Geometry: final body of the model. Coordinates: model frame, mm. A direction names the side the tool comes from. Round coordinates to 2 decimals unless told otherwise and drop trailing zeros. Loops run counter-clockwise (first coordinate to the right, second up) from the corner with the lowest first, then second, coordinate; pieces in that order, holes last. Notation, with made-up numbers: M 19.5,65.25 L 69.5,65.25 A21 cw 69.5,98.25 Z; hole C 50,64 d2. An arc over 180 degrees is marked long. Write each question's results on one line, items separated by ' | '.
```python
from build123d import *

# Parameters (mm, degrees)
F1_DEPTH = 10
F2_SIZE  = 9.99999


# Not quite as in the source:
# - a fillet or chamfer is up to 0.001 mm smaller than in the source, because OpenCascade refuses the exact size


with BuildPart() as f1:
    # F0 (on Front) → F1 (new body)
    with BuildSketch(Plane.XZ):
        Polygon((70, -108.8627894558), (70, 125), (-70, 125), (-70, -125), (-54, -125), (-45, -109.0002581477), (45.5037690699, -109.0002581477), (54, -125), (70, -125), align=None)
    extrude(amount=F1_DEPTH)

    # F2 (size 10 in the source; OpenCascade refuses exactly that, so slightly less here)
    f2_edges = [f1.edges().sort_by_distance(p)[0] for p in [
        (-70, 0, 0),
        (70, 0, 0),
    ]]
    chamfer(f2_edges, length=F2_SIZE)


solid = f1.part
```
1. Section B-B (y = -5.75). Output: boundary loops of the cut face in (x, z).
Answer key:
outline: M -65.75,-125 L -54,-125 L -45,-109 L 45.5,-109 L 54,-125 L 65.75,-125 L 65.75,125 L -65.75,125 Z
2. Section C-C (x = -22). Output: boundary loops of the cut face in (y, z), then the cut area to 3 significant figures.
Answer key:
outline: M -10,-109 L 0,-109 L 0,125 L -10,125 Z | area: 2,340 mm²
3. Access query for faces 1 (the face through (49.7, -4.9, -116.9)), 2 (the face through (-1, -10, 2)). Directions: +Z, -Z, +X, -X, +Y, -Y. A direction counts if a zero-diameter tool reaches every point of the face in a straight line with its end or side. Return the directions, or none.
Answer key:
face 1: -Z, +Y, -Y | face 2: +Z, -Z, +X, -X, -Y
4. Pin query (flat end, axial travel): P1, Ø4, axis at y = -5.5, z = -5, coming from the +X side; P2, Ø6, axis at x = -32, y = -4.5, coming from the -Z side; P3, Ø3, axis at y = -4.5, z = -50, coming from the +X side. Return the tip coordinate at first contact, or that it passes through.
Answer key:
P1: stops at x = 67.5 | P2: stops at z = -109 | P3: stops at x = 66
5. Draft query along X for faces 3 (the face through (65, -5, -2)), 4 (the face through (-1, 0, 2)), 5 (the face through (-49.56, -4.93, -117.11)). Return one class per face: pulls with the +X half, pulls with the -X half, needs draft (parallel to the pull), parting line crosses it, or undercut.
Answer key:
face 3: pulls with the +X half | face 4: needs draft | face 5: undercut
6. Ray query, probe 1 along Z at (x, y) = (44, -9.5); probe 2 along Y at (x, z) = (-63.5, 99.5); probe 3 along X at (y, z) = (-3.5, -90). Return the intervals inside material, ascending.
Answer key:
probe 1: z = -109 to 125 | probe 2: y = -10 to -3.5 | probe 3: x = -63.5 to 63.5
